Job drawing, mm, ordinate dimensions from the low corner. One solid piece. Give positions to 0.01 mm unless a question says otherwise; leave off trailing zeros. Write each loop counter-clockwise with the first axis right and the second up, starting at its lowest first coordinate (ties: lowest second). Pieces come first, ordered by that corner, then holes. Notation, with made-up numbers: M 29,5.25 L 57,5.25 A23 cw 57,43.25 Z; hole C 13.5,53.25 d9. An arc over 180 degrees is marked long. Use a Markdown table: item, result.
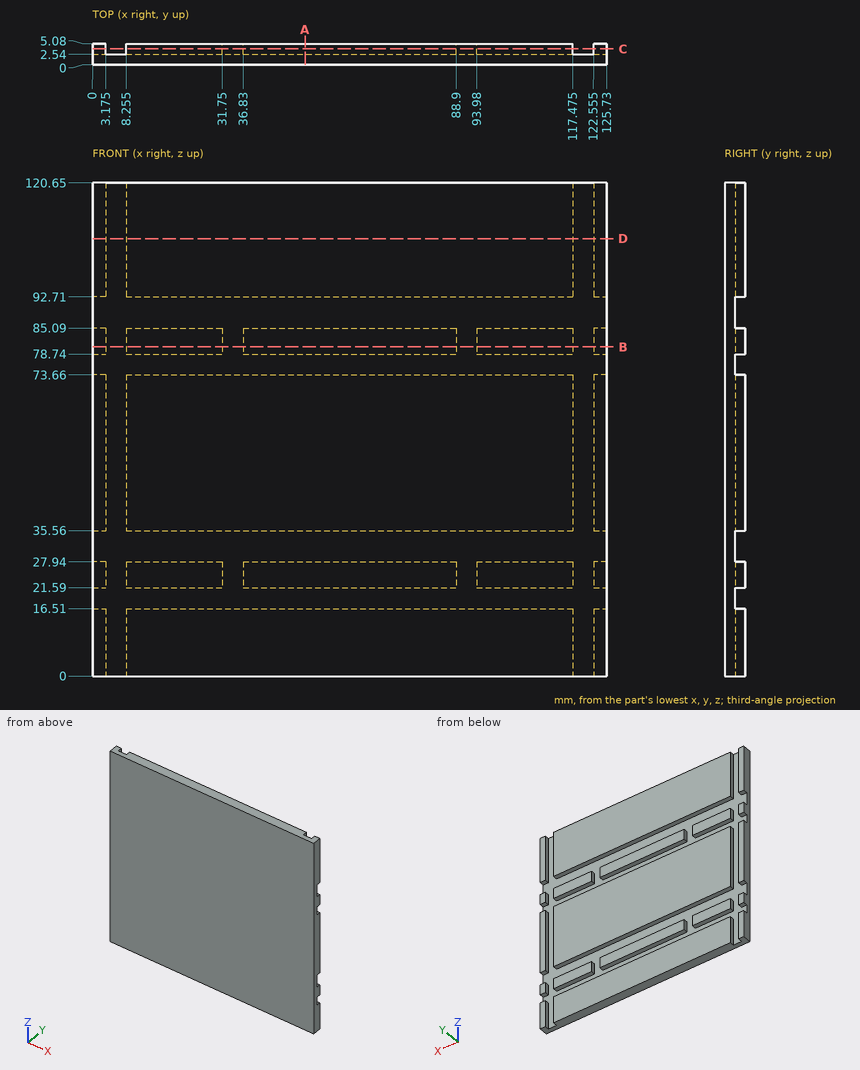
1. Drop flat-ended pins along their axis: P1, Ø1, axis at x = 96, y = 3, coming from the -Z side; P2, Ø2, axis at y = 4.5, z = 76.5, coming from the +X side. Give the stop position or say it passes through.
Findings below:
| item | result |
|---|---|
| P1 | z = 0 |
| P2 | through |
2. Drill centre lines: L1, parallel to X at y = 3.85, z = 41 (3 decimals); L2, parallel to Z at x = 74, y = 4.85; L3, parallel to Z at x = 89.5, y = 3. Where is each one in solid material? Low to high.
Findings below:
| item | result |
|---|---|
| L1 | 0 to 3.175, 8.255 to 117.475, 122.555 to 125.73 |
| L2 | 0 to 16.51, 21.59 to 27.94, 35.56 to 73.66, 78.74 to 85.09, 92.71 to 120.65 |
| L3 | 0 to 16.51, 35.56 to 73.66, 92.71 to 120.65 |
3. Cut at B-B, the plane z = 80.5. Give the cut face in (x, y) (3 decimals).
Findings below:
| item | result |
|---|---|
| outline | M 0,0 L 125.73,0 L 125.73,5.08 L 122.555,5.08 L 122.555,2.54 L 117.475,2.54 L 117.475,5.08 L 93.98,5.08 L 93.98,2.54 L 88.9,2.54 L 88.9,5.08 L 36.83,5.08 L 36.83,2.54 L 31.75,2.54 L 31.75,5.08 L 8.255,5.08 L 8.255,2.54 L 3.175,2.54 L 3.175,5.08 L 0,5.08 Z |
4. Cut at A-A, the plane x = 52. Give the cut face in (y, z), then the cut area to 3 significant figures.
Findings below:
| item | result |
|---|---|
| outline | M 0,0 L 5.08,0 L 5.08,16.51 L 2.54,16.51 L 2.54,21.59 L 5.08,21.59 L 5.08,27.94 L 2.54,27.94 L 2.54,35.56 L 5.08,35.56 L 5.08,73.66 L 2.54,73.66 L 2.54,78.74 L 5.08,78.74 L 5.08,85.09 L 2.54,85.09 L 2.54,92.71 L 5.08,92.71 L 5.08,120.65 L 0,120.65 Z |
| area | 548 mm2 |
5. Cut at D-D, the plane z = 107. Give the cut face in (x, y) (3 decimals).
Findings below:
| item | result |
|---|---|
| outline | M 0,0 L 125.73,0 L 125.73,5.08 L 122.555,5.08 L 122.555,2.54 L 117.475,2.54 L 117.475,5.08 L 8.255,5.08 L 8.255,2.54 L 3.175,2.54 L 3.175,5.08 L 0,5.08 Z |
6. Cut at C-C, the plane y = 3.9. State how many separate pieces and enclosed holes the cut face has, then the cut area to 3 significant figures.
Findings below:
| item | result |
|---|---|
| separate pieces | 19 |
| enclosed holes | 0 |
| area | 10,900 mm2 |
